Autodesk Inventor part; units mm, degrees
ref_plane "Work Plane1" through (0, 0, -23) normal (0, 0, 1) x (1, 0, 0)
ref_plane "Work Plane2" through (0, 0, -2) normal (0, 0, 1) x (1, 0, 0)
ref_plane "YZ Plane" through (0, 0, 0) normal (1, 0, 0) x (0, 1, 0)
sketch "Sketch2" plane through (0, 0, 0) normal (0, 0, 1) x (1, 0, 0)
  circle A0 centre (0, 0) radius 2.75
  dimension "d0" = 5.5
extrude "Extrusion1" add sketch "Sketch2" against normal blind 14.5
fillet "Fillet1" radius 2.75 1 edges at (-2.75, 0, -14.5)
sketch "Sketch3" plane through (0, 0, 0) normal (0, 1, 0) x (-1, 0, 0)
  line L0 (2.75, 0) -> (-2.75, 0) construction
  line L1 (-2.75, -11.75) -> (2.75, -11.75) construction
  arc A0 (-3.4924, -19.2699) -> (3.4924, -19.2699) centre (0, -19.5) ccw
  line L2 (3.4924, -19.2699) -> (2.75, -8)
  line L3 (-3.4924, -19.2699) -> (-2.75, -8)
  line L4 (0, -27.6) -> (0, 4.6) construction
  line L5 (2.75, 0) -> (2.75, -11.75) construction
  line L6 (-2.75, 0) -> (-2.75, -11.75) construction
  line L7 (-2.75, -8) -> (2.75, -8)
  point P0 (0, 0)
  dimension "d4" = 7
  dimension "d5" = 8
  dimension "d6" = 19.5
  dimension "d7" = 8
extrude "Extrusion2" add sketch "Sketch3" along normal mid plane 2.5
sketch "Sketch4" plane through (0, 0, 0) normal (0, 1, 0) x (-1, 0, 0)
  arc A0 (-3.4924, -19.2699) -> (3.4924, -19.2699) centre (0, -19.5) ccw construction
  arc A1 (-2.4, -19.5) -> (2.4, -19.5) centre (0, -19.5) ccw
  line L0 (2.4, -19.5) -> (-2.4, -19.5)
  point P0 (0, 0)
  dimension "d10" = 4.8
revolve "Revolution1" cut sketch "Sketch4" angle 360 about axis through (-2.4, 0, -19.5) along (1, 0, 0)
sketch "Sketch5" plane through (0, 0, 0) normal (0, 0, 1) x (1, 0, 0)
  circle A0 centre (0, 0) radius 1.5
  dimension "d12" = 3
extrude "Extrusion3" cut sketch "Sketch5" against normal blind 12
thread "Thread1"
ref_plane "Work Plane1" through (0, 0, -23) normal (0, 0, 1) x (1, 0, 0)
sketch "Sketch6" plane through (0, 0, -23) normal (0, 0, 1) x (1, 0, 0)
  line L0 (-4.9, 0) -> (4.9, 0) construction
  line L1 (0, -3.85) -> (0, 3.85) construction
  line L2 (1.25, 1.25) -> (-1.25, 1.25)
  line L3 (-1.25, 1.25) -> (-1.25, -1.25)
  line L4 (-1.25, -1.25) -> (1.25, -1.25)
  line L5 (1.25, -1.25) -> (1.25, 1.25)
  point P0 (0, 0)
  dimension "d17" = 2.5
  dimension "d18" = 2.5
extrude "Extrusion4" add sketch "Sketch6" against normal blind 2
sketch "Sketch7" plane through (0, 0, -23) normal (0, 0, 1) x (1, 0, 0)
  line L0 (-1.25, -1.25) -> (-1.25, 1.25) construction
  line L1 (-1.25, 1.25) -> (1.25, 1.25) construction
  line L2 (1.25, 1.25) -> (1.25, -1.25) construction
  line L3 (1.25, -1.25) -> (-1.25, -1.25) construction
  line L4 (-1.25, 1.25) -> (1.25, 1.25)
  line L5 (1.25, 1.25) -> (1.25, -1.25)
  line L6 (1.25, -1.25) -> (-1.25, -1.25)
  line L7 (-1.25, -1.25) -> (-1.25, 1.25)
  point P0 (0, 0)
extrude "Extrusion5" add sketch "Sketch7" along normal up to surface
ref_plane "Work Plane2" through (0, 0, -2) normal (0, 0, 1) x (1, 0, 0)
sketch "Sketch8" plane through (0, 0, -2) normal (0, 0, 1) x (1, 0, 0)
  arc A0 (2.4495, 1.25) -> (-2.4495, 1.25) centre (0, 0) ccw construction
  circle A1 centre (0, 0) radius 2.75
  line L0 (0, -3.85) -> (0, 3.85) construction
  line L1 (-4.9, 0) -> (4.9, 0) construction
  line L2 (-1, 2.5617) -> (0, 3.5)
  line L3 (1, 2.5617) -> (0, 3.5)
  dimension "d24" = 3.5
  dimension "d25" = 2
extrude "Extrusion6" add sketch "Sketch8" against normal blind 9 contours A1 L2 L3
mirror "Mirror1" about plane through (0, 0, 0) normal (0, 1, 0) of "Extrusion6"
properties part number "Rotule_M3" material "POM"
Verification items for the finished model (mm, model axes). A direction names the side the tool comes from. Coordinates: 2 decimals unless noted, no trailing zeros. Order: outer loops, then holes, each group sorted by start corner. A loop starts at its lowest first (then second) coordinate and runs counter-clockwise, first axis right, second up. Notation, with made-up numbers: (-39, 64.5) -> (-3, 64.5) arc R22 ccw to (-3, 99.5) -> close; hole circle Ø8 at (-20.5, 24). An arc over 180 degrees is marked (long way). Answer as CSV lines item,"result". Start each with the question number.
1) Cross-section at D-D, the plane z = -10.25. Record the boundary of the cut face in (x, y).
2) Cross-section at B-B, the plane z = -17.75. Record the boundary of the cut face in (x, y), then the cut area to 3 significant figures.
3) Material ranges on L1, parallel to Y at x = 0.25, z = -17; L2, parallel to Z at x = -2, y = -0.5; L3, parallel to Z at x = -1.5, y = -1, recorded low to high. Write a range as [from, to].
4) Set-up check for faces 1 (the face through (-0.51, 3.02, -6.44)), 2 (the face through (1.25, 0, -24)), 3 (the face through (-1.25, 0, -24)): record each of +Z, -Z, +X, -X, +Y, -Y from which the full face is reachable in a straight line by a thin tool's end or side.
5) Cross-section at A-A, the plane y = 0.75. Record the boundary of the cut face in (x, z).
6) Gauge pin test, flat ends, axial feed: pin 1 Ø2 at (y, z) = (1, -8) entering from -X; pin 2 Ø3.5 at (x, z) = (-1, -13) entering from +Y; pin 3 Ø1 at (y, z) = (1, -8.5) entering from +X. Record the tip position at first contact, or that the pin passes through.
7) Release check for a two-part mould opening along X. For faces 4 (the face through (-2.964, -0.018, -21.362)), 5 (the face through (0, 3, -2)), 6 (the face through (-1.5, 0.07, -5.92)) record: released by +X, released by -X, zero draft, split by the parting line, or undercut.
8) Cross-section at C-C, the plane x = 0.25. Record the boundary of the cut face in (y, z).
Conclusion:
1,outline,"(-2.9, -1.25) -> (-2.45, -1.25) arc R2.75 ccw to (-1, -2.56) -> (0, -3.5) -> (1, -2.56) arc R2.75 ccw to (2.45, -1.25) -> (2.9, -1.25) -> (2.9, 1.25) -> (2.45, 1.25) arc R2.75 ccw to (1, 2.56) -> (0, 3.5) -> (-1, 2.56) arc R2.75 ccw to (-2.45, 1.25) -> (-2.9, 1.25) -> close; hole circle Ø3 at (0, 0)"
2,outline,"(-3.39, -1.25) -> (-1.07, -1.25) arc R1.64 cw to (-1.07, 1.25) -> (-3.39, 1.25) -> close; (1.07, -1.25) -> (3.39, -1.25) -> (3.39, 1.25) -> (1.07, 1.25) arc R1.64 cw to start"
2,area,"9.63 mm²"
3,L1,"y = [-1.25, 1.25]"
3,L2,"z = [-22.37, -20.73], [-18.27, 0]"
3,L3,"z = [-22.66, -21.08], [-17.92, 0]"
4,face 1,"+Z, -Z, -X, +Y"
4,face 2,"-Z, +X, +Y, -Y"
4,face 3,"-Z, -X, +Y, -Y"
5,outline,"(-3.49, -19.27) arc R3.5 ccw to (-1.25, -22.77) -> (-1.25, -25) -> (1.25, -25) -> (1.25, -22.77) arc R3.5 ccw to (3.49, -19.27) -> (2.75, -8) -> (2.65, -8) -> (2.65, 0) -> (1.3, 0) -> (1.3, -12) -> (-1.3, -12) -> (-1.3, 0) -> (-2.65, 0) -> (-2.65, -8) -> (-2.75, -8) -> close; hole circle Ø4.56 at (0, -19.5)"
6,pin 1,"stops at x = -2.82"
6,pin 2,"stops at y = 2.75"
6,pin 3,"stops at x = 2.82"
7,face 4,"released by -X"
7,face 5,"zero draft"
7,face 6,"undercut"
8,outline,"(-3.27, -11) -> (-2.74, -11) -> (-2.74, -11.75) arc R2.74 ccw to (-1.25, -14.19) -> (-1.25, -17.47) arc R2.39 cw to (1.25, -17.47) -> (1.25, -14.19) arc R2.74 ccw to (2.74, -11.75) -> (2.74, -11) -> (3.27, -11) -> (3.27, -2) -> (2.74, -2) -> (2.74, 0) -> (1.48, 0) -> (1.48, -12) -> (-1.48, -12) -> (-1.48, 0) -> (-2.74, 0) -> (-2.74, -2) -> (-3.27, -2) -> close; (-1.25, -25) -> (1.25, -25) -> (1.25, -21.53) arc R2.39 cw to (-1.25, -21.53) -> close"
